Could you check a few things on this drawing? It's one solid part, dimensions in mm from its lowest x, y, z. Round coordinates to 2 decimals unless told otherwise and drop trailing zeros. Order: outer loops, then holes, each group sorted by start corner. A loop starts at its lowest first (then second) coordinate and runs counter-clockwise, first axis right, second up. Notation, with made-up numbers: M 44,-15 L 92,-15 A12 ccw 92,7 Z; hole C 21.25,-12 d10. An arc over 180 degrees is marked long. Answer as CSV lines item,"result". Start each with the question number.
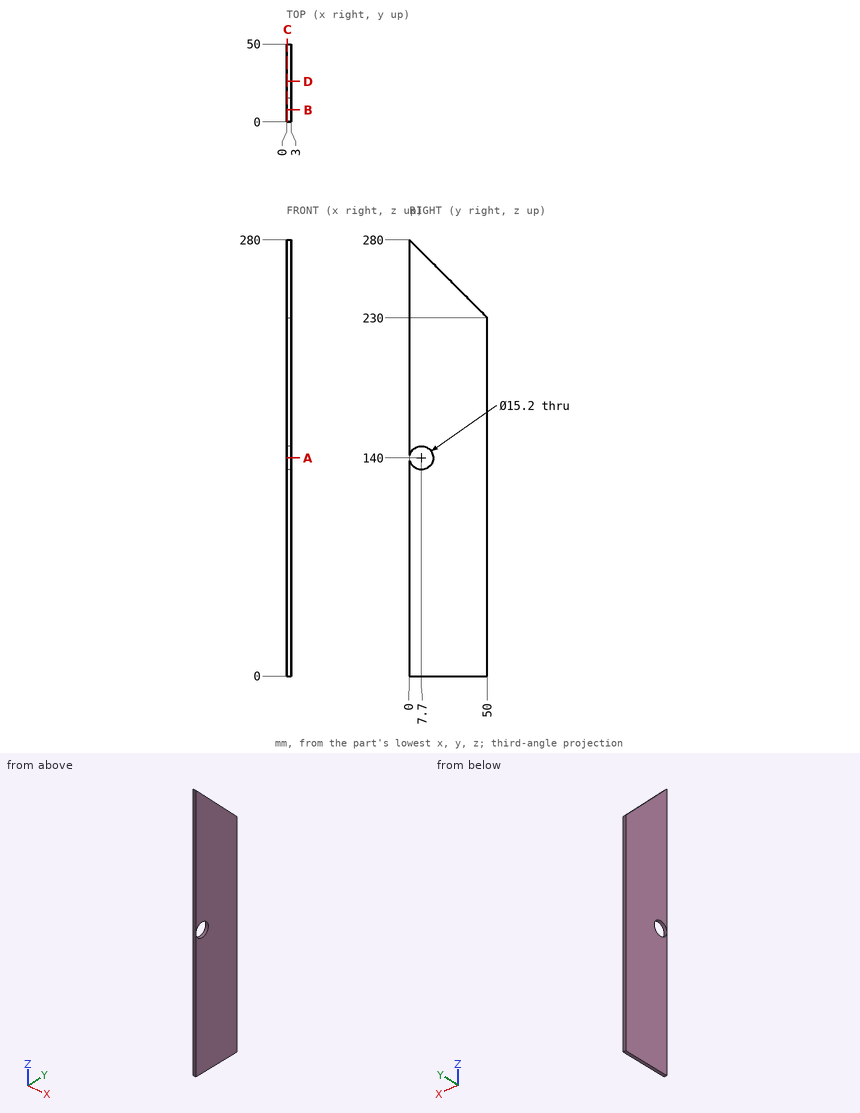
Item 1: If we section it at C-C on x = 0.45: Please give me the cut outline in (y, z), and give its area (3 significant figures).
Item 2: If I drill on line 1 along Z through (x, y) = (2.1, 9.5); line 2 along Z through (x, y) = (2.7, 16); line 3 along Z through (x, y) = (2.25, 36), over which ranges is the centre line in solid material (lowest first)?
Item 3: If we section it at B-B on y = 7.7: Please give me the cut outline in (x, z).
Item 4: If we section it at D-D on y = 26: Please give me the cut outline in (x, z).
Item 5: If we section it at A-A on z = 140: Please give me the cut outline in (x, y).
Item 6: For P1, Ø5, axis at y = 40.5, z = 174.5, coming from the -X side; P2, Ø1, axis at x = 1.5, y = 13.5, coming from the +Z side; P3, Ø1.5, axis at x = 2.5, y = 40, coming from the +Z side; P4, Ø13.5, axis at y = 7.7, z = 140, coming from the -X side, each with a flat end and sliding along its axis, tell me the tip position at first contact or that it passes through.
Geometry says:
1,outline,"M 0,0 L 50,0 L 50,230 L 0,280 Z; hole C 7.7,140 d15.2"
1,area,"12,600 mm²"
2,line 1,"0 to 132.62, 147.38 to 270.5"
2,line 2,"0 to 264"
2,line 3,"0 to 244"
3,outline,"M 0,0 L 3,0 L 3,132.4 L 0,132.4 Z; M 0,147.6 L 3,147.6 L 3,272.3 L 0,272.3 Z"
4,outline,"M 0,0 L 3,0 L 3,254 L 0,254 Z"
5,outline,"M 0,0 L 3,0 L 3,0.1 L 0,0.1 Z; M 0,15.3 L 3,15.3 L 3,50 L 0,50 Z"
6,P1,"x = 0"
6,P2,"z = 267"
6,P3,"z = 240.75"
6,P4,"through"
